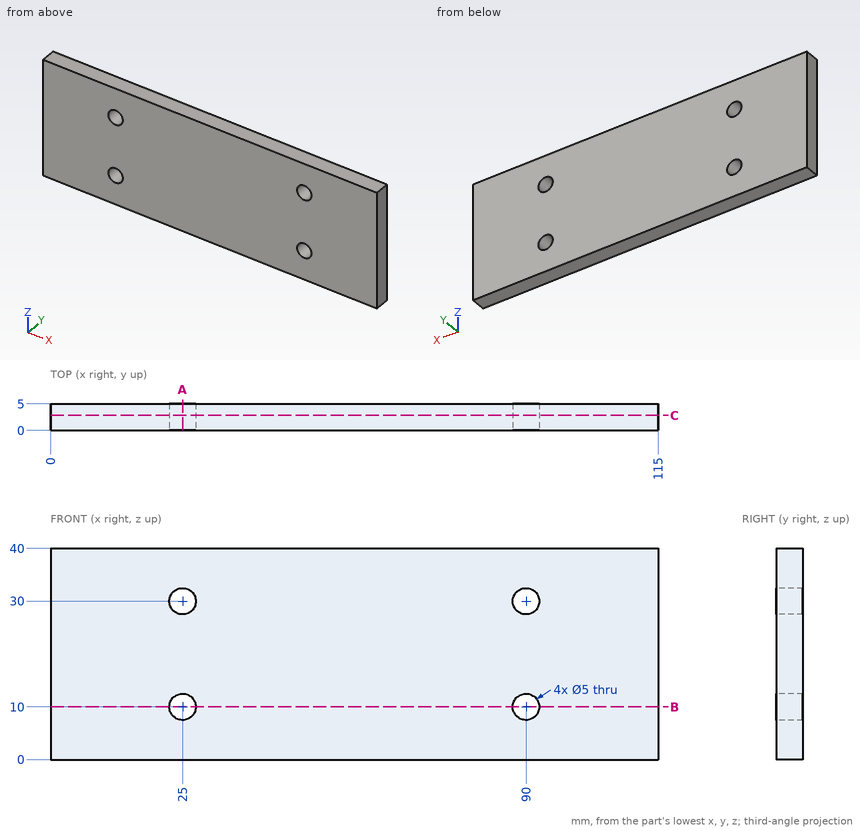
Answer from the drawing. Dimensions are ordinates in mm from the lowest x, y and z of the part. Coordinates: 2 decimals unless noted, no trailing zeros. Loops run counter-clockwise (first coordinate to the right, second up) from the corner with the lowest first, then second, coordinate; pieces in that order, holes last.
1) Section C-C (y = 2.85) is taken. Give the vertices of the cut face in (x, z).
Results:
outline: (0, 0) - (115, 0) - (115, 40) - (0, 40) - close; hole circle Ø5 at (25, 10); hole circle Ø5 at (25, 30); hole circle Ø5 at (90, 10); hole circle Ø5 at (90, 30)
2) Consider probe 1 along X at (y, z) = (3.15, 30); probe 2 along Z at (x, y) = (25, 2.85); probe 3 along Z at (x, y) = (92, 4.7). Determine where each line is inside the solid, lowest interval first.
Results:
probe 1: x = 0 to 22.5, 27.5 to 87.5, 92.5 to 115
probe 2: z = 0 to 7.5, 12.5 to 27.5, 32.5 to 40
probe 3: z = 0 to 8.5, 11.5 to 28.5, 31.5 to 40
3) Section A-A (x = 25) is taken. Give the vertices of the cut face in (y, z).
Results:
outline: (0, 0) - (5, 0) - (5, 7.5) - (0, 7.5) - close; (0, 12.5) - (5, 12.5) - (5, 27.5) - (0, 27.5) - close; (0, 32.5) - (5, 32.5) - (5, 40) - (0, 40) - close
4) Section B-B (z = 10) is taken. Give the vertices of the cut face in (x, y), plus the area to 3 significant figures.
Results:
outline: (0, 0) - (22.5, 0) - (22.5, 5) - (0, 5) - close; (27.5, 0) - (87.5, 0) - (87.5, 5) - (27.5, 5) - close; (92.5, 0) - (115, 0) - (115, 5) - (92.5, 5) - close
area: 525 mm2
